Autodesk Fusion 360 part; units mm, degrees
sketch "Boceto1" plane through (0, 0, 0) normal (0, 1, 0) x (1, 0, 0)
  circle A0 centre (70, 0) radius 45
extrude "Extruir2" add sketch "Boceto1" along normal blind 14.2 makes body 1
sketch "Boceto2" plane through (0, 0, 0) normal (0, 1, 0) x (1, 0, 0)
  circle A0 centre (70, -35) radius 6.25
  circle A1 centre (35, 0) radius 6.25
  circle A2 centre (70, 35) radius 6.25
  circle A3 centre (105, 0) radius 6.25
extrude "Extruir3" cut sketch "Boceto2" along normal blind 15 bodies 1
sketch "Boceto3" plane through (0, 0, 0) normal (0, 1, 0) x (1, 0, 0)
  circle A0 centre (70, 0) radius 19
  circle A1 centre (70, 0) radius 24
  line L0 (70, -45) -> (70, -24)
  line L1 (70, -19) -> (70, 19)
  line L2 (70, 24) -> (70, 45)
  line L3 (25, 0) -> (46, 0)
  line L4 (51, 0) -> (89, 0)
  line L5 (94, 0) -> (115, 0)
extrude "Extruir5" add sketch "Boceto3" against normal blind 44.2 bodies 1
sketch "Boceto7" plane through (0, 0, 0) normal (0, 1, 0) x (1, 0, 0)
  circle A0 centre (-25, 0) radius 25
  circle A1 centre (-25, 0) radius 19
extrude "Extruir6" add sketch "Boceto7" against normal blind 30 separate body makes body 2
delete_face "SuprimirCaras2" 1 faces at (93.8807, -29.4667, 2.3896) on bodies 1
sketch "Boceto8" plane through (0, 0, 0) normal (0, 1, 0) x (1, 0, 0)
  circle A0 centre (70, 0) radius 15
  circle A1 centre (70, 0) radius 20
extrude "Extruir7" add sketch "Boceto8" against normal blind 44.2 bodies 1
move_body "Alinear1" bodies 2 to x (1, 0, 0) y (0, 1, 0) z (0, 0, 1) at (95, -14.2, 0)
move_body "Desplazar1" bodies 2 to x (1, 0, 0) y (0, 1, 0) z (0, 0, 1) at (0, -30, 0)
combine "Combinar1" operation add target body 1 tool bodies 2
Build history of the part. All positions in model axes, mm. A direction names the side the tool comes from. Round coordinates to 2 decimals unless told otherwise and drop trailing zeros. Loops run counter-clockwise (first coordinate to the right, second up) from the corner with the lowest first, then second, coordinate; pieces in that order, holes last.
Item 1: Drill centre lines: line 1 along X through (y, z) = (11.5, 0); line 2 along Z through (x, y) = (69.5, -19); line 3 along Z through (x, y) = (70, -59). Where is each one in solid material? Low to high.
Item 2: Saw through at B-B (z = 35). List the corners of the cut face in (x, y).
Item 3: Pin check, flat tips, straight feed: P1, Ø14.5, axis at x = 70, z = -35, coming from the -Y side; P2, Ø24, axis at x = 74.5, z = 3.5, coming from the -Y side; P3, Ø2, axis at x = 87.5, y = -13.5, coming from the -Z side; P4, Ø11, axis at x = 35, z = 0, coming from the -Y side. Stop position of each tip, or through.
Item 4: Saw through at D-D (y = -60). List the corners of the cut face in (x, z).
Item 5: Saw through at C-C (x = 105). List the corners of the cut face in (y, z).
Item 6: Two-plate mould, pull along Z, no slides. Class faces 4 (the face through (45.024, -58.99, -1.099)), 5 (the face through (79, 0, 19)), 6 (the face through (55.015, -21.791, -0.66)): released by +Z, released by -Z, zero draft, split by the parting line, or undercut.
Item 7: Which spindle directions (+Z, -Z, +X, -X, +Y, -Y) get a long thin tool onto all of the face, cutting with end or side? Do faces 1 (the face through (59, -44.2, -17)), 2 (the face through (75.96, 7, -33.12)), 3 (the face through (70, 0, 0)). Say none if no direction does.
Item 8: Saw through at A-A (x = 70). List the corners of the cut face in (y, z).
Worked answers:
1. line 1: x = 25 to 28.75, 41.25 to 98.75, 111.25 to 115
1. line 2: z = -19.99 to -14.99, 14.99 to 19.99
1. line 3: z = -25 to -19, 19 to 25
2. outline: (41.72, 0) - (63.75, 0) - (63.75, 14.2) - (41.72, 14.2) - close; (76.25, 0) - (98.28, 0) - (98.28, 14.2) - (76.25, 14.2) - close
3. P1: stops at y = 0
3. P2: stops at y = -44.2
3. P3: stops at z = -11.3
3. P4: passes through
4. outline: circle Ø50 at (70, 0); hole circle Ø38 at (70, 0)
5. outline: (0, -28.28) - (14.2, -28.28) - (14.2, -6.25) - (0, -6.25) - close; (0, 6.25) - (14.2, 6.25) - (14.2, 28.28) - (0, 28.28) - close
6. face 4: split by the parting line
6. face 5: zero draft
6. face 6: undercut
7. face 1: none
7. face 2: +Y, -Y
7. face 3: -Y
8. outline: (-74.2, -25) - (-44.2, -25) - (-44.2, -20) - (0, -20) - (0, -28.75) - (14.2, -28.75) - (14.2, 28.75) - (0, 28.75) - (0, 20) - (-44.2, 20) - (-44.2, 25) - (-74.2, 25) - (-74.2, 19) - (-44.2, 19) - (-44.2, 15) - (0, 15) - (0, -15) - (-44.2, -15) - (-44.2, -19) - (-74.2, -19) - close; (0, -45) - (14.2, -45) - (14.2, -41.25) - (0, -41.25) - close; (0, 41.25) - (14.2, 41.25) - (14.2, 45) - (0, 45) - close
